from build123d import *

# Parameters (mm, degrees)
SKETCH1_W           = 45
SKETCH1_H           = 70
BOSS_EXTRUDE1_DEPTH = 20
SKETCH2_W           = 42
SKETCH2_H           = 67
CUT_EXTRUDE1_DEPTH  = 86.586213843
CUT_EXTRUDE2_DEPTH  = 84.150466024
CUT_EXTRUDE3_DEPTH  = 85.047605558
CHAMFER1_SIZE       = 2
FILLET1_R           = 3
FILLET2_R           = 6


with BuildPart() as part:
    # Sketch1 → Boss-Extrude1 (new body)
    with BuildSketch(Plane(origin=(20, 0, 0), x_dir=(0, 0, -1), z_dir=(1, 0, 0))):
        with Locations((22.5, 35)):
            Rectangle(SKETCH1_W, SKETCH1_H)
    extrude(amount=-BOSS_EXTRUDE1_DEPTH)

    # Sketch2 → Cut-Extrude1 (cut, through all)
    with BuildSketch(Plane.ZY):
        with Locations((-24, 36.5)):
            Rectangle(SKETCH2_W, SKETCH2_H)
    extrude(amount=-CUT_EXTRUDE1_DEPTH, mode=Mode.SUBTRACT)

    # Sketch3 → Cut-Extrude2 (cut, through all)
    with BuildSketch(Plane(origin=(0, 3, 0), x_dir=(-1, 0, 0), z_dir=(0, 1, 0))):
        with BuildLine():
            Line((-5.5, -33), (-5.5, -13))
            ThreePointArc((-5.5, -13), (-10, -8.5), (-14.5, -13))
            Line((-14.5, -13), (-14.5, -33))
            ThreePointArc((-14.5, -33), (-10, -37.5), (-5.5, -33))
        make_face()
    extrude(amount=-CUT_EXTRUDE2_DEPTH, mode=Mode.SUBTRACT)

    # Sketch4 → Cut-Extrude3 (cut, through all)
    with BuildSketch(Plane(origin=(0, 0, -3), x_dir=(-1, 0, 0), z_dir=(0, 0, -1))):
        with BuildLine():
            Line((-14.5, 60), (-14.5, 20))
            ThreePointArc((-14.5, 20), (-10, 15.5), (-5.5, 20))
            Line((-5.5, 20), (-5.5, 60))
            ThreePointArc((-5.5, 60), (-10, 64.5), (-14.5, 60))
        make_face()
    extrude(amount=-CUT_EXTRUDE3_DEPTH, mode=Mode.SUBTRACT)

    # Chamfer1
    chamfer1_edges = [part.edges().sort_by_distance(p)[0] for p in [
        (0, 1.5, -45),
        (20, 70, -1.5),
        (0, 70, -1.5),
        (20, 1.5, -45),
    ]]
    chamfer(chamfer1_edges, length=CHAMFER1_SIZE)

    # Fillet1
    fillet1_edges = [part.edges().sort_by_distance(p)[0] for p in [
        (10, 3, -3),
    ]]
    fillet(fillet1_edges, radius=FILLET1_R)

    # Fillet2
    fillet2_edges = [part.edges().sort_by_distance(p)[0] for p in [
        (10, 0, 0),
    ]]
    fillet(fillet2_edges, radius=FILLET2_R)


solid = part.part
Geometry check sheet. Reference: the model listing, model coordinates, mm. A direction names the side the tool comes from. Round coordinates to 2 decimals unless told otherwise and drop trailing zeros. Write each loop counter-clockwise with the first axis right and the second up, starting at its lowest first coordinate (ties: lowest second). Pieces come first, ordered by that corner, then holes. Notation, with made-up numbers: (-17, 27.5) -> (15, 27.5) arc R17 ccw to (15, 35.5) -> close; hole circle Ø8 at (16, 6). An arc over 180 degrees is marked (long way). One line per item, written item: value. Start each with the question number.
(1) Scan lines: line 1 (X direction, y = 37.5, z = -2.5); line 2 (Y direction, x = 5.25, z = -25); line 3 (Z direction, x = 16, y = 8). Record each from-to range of solid material in increasing order. Write a range as [from, to].
(2) Cross-section at D-D, the plane x = 16. Record the cut outline in (y, z), and give its area (3 significant figures).
(3) Draft check along X on faces 5 (the flat face through (1, 1, -44)), 6 (the flat face through (5, 38, -3)), 7 (the flat face through (14.5, 2, -23)), 8 (the cylindrical face through (9.9, 1.5, -8.5)). Enter one of: +X half, -X half, draft (parallel to the pull), parting line (faces both ways), or undercut.
(4) Cross-section at C-C, the plane y = 43. Record the cut outline in (x, z), and give its area (3 significant figures).
(5) Cross-section at B-B, the plane z = -28. Record the cut outline in (x, y), and give its area (3 significant figures).
(6) Access from +Z, -Z, +X, -X, +Y, -Y to the whole of each face (thin tool, end or side, straight path). Record for faces 1 (the cylindrical face through (10.1, 1.5, -37.5)), 2 (the cylindrical face through (9.9, 64.5, -1.5)), 3 (the flat face through (1, 69, -1)), 4 (the flat face through (5, 3, -26)).
(7) Cross-section at A-A, the plane x = 10. Record the cut outline in (y, z), and give its area (3 significant figures).
(8) Go/stop test with flat-tipped pins: pin 1 Ø10 at (x, z) = (9.5, -21) entering from -Y; pin 2 Ø3 at (x, y) = (2, 61) entering from -Z; pin 3 Ø2 at (x, z) = (4, -24) entering from +Y. Record where each tip stops, or that it passes through.
Answer:
1. line 1: [0, 5.5], [14.5, 20]
1. line 2: [0, 3]
1. line 3: [-3, 0]
2. outline: (0, -45) -> (3, -45) -> (3, -6) arc R3 cw to (6, -3) -> (70, -3) -> (70, 0) -> (6, 0) arc R6 ccw to (0, -6) -> close
2. area: 330 mm²
3. face 5: -X half
3. face 6: draft
3. face 7: undercut
3. face 8: undercut
4. outline: (0, -3) -> (5.5, -3) -> (5.5, 0) -> (0, 0) -> close; (14.5, -3) -> (20, -3) -> (20, 0) -> (14.5, 0) -> close
4. area: 33.0 mm²
5. outline: (0, 0) -> (5.5, 0) -> (5.5, 3) -> (0, 3) -> close; (14.5, 0) -> (20, 0) -> (20, 3) -> (14.5, 3) -> close
5. area: 33.0 mm²
6. face 1: +Y, -Y
6. face 2: +Z, -Z
6. face 3: +Z, -Z, -X, +Y
6. face 4: -Z, +X, -X, +Y
7. outline: (0, -45) -> (3, -45) -> (3, -37.5) -> (0, -37.5) -> close; (0, -8.5) -> (3, -8.5) -> (3, -6) arc R3 cw to (6, -3) -> (15.5, -3) -> (15.5, 0) -> (6, 0) arc R6 ccw to (0, -6) -> close; (64.5, -3) -> (70, -3) -> (70, 0) -> (64.5, 0) -> close
7. area: 96.2 mm²
8. pin 1: y = 0
8. pin 2: z = -3
8. pin 3: y = 3
